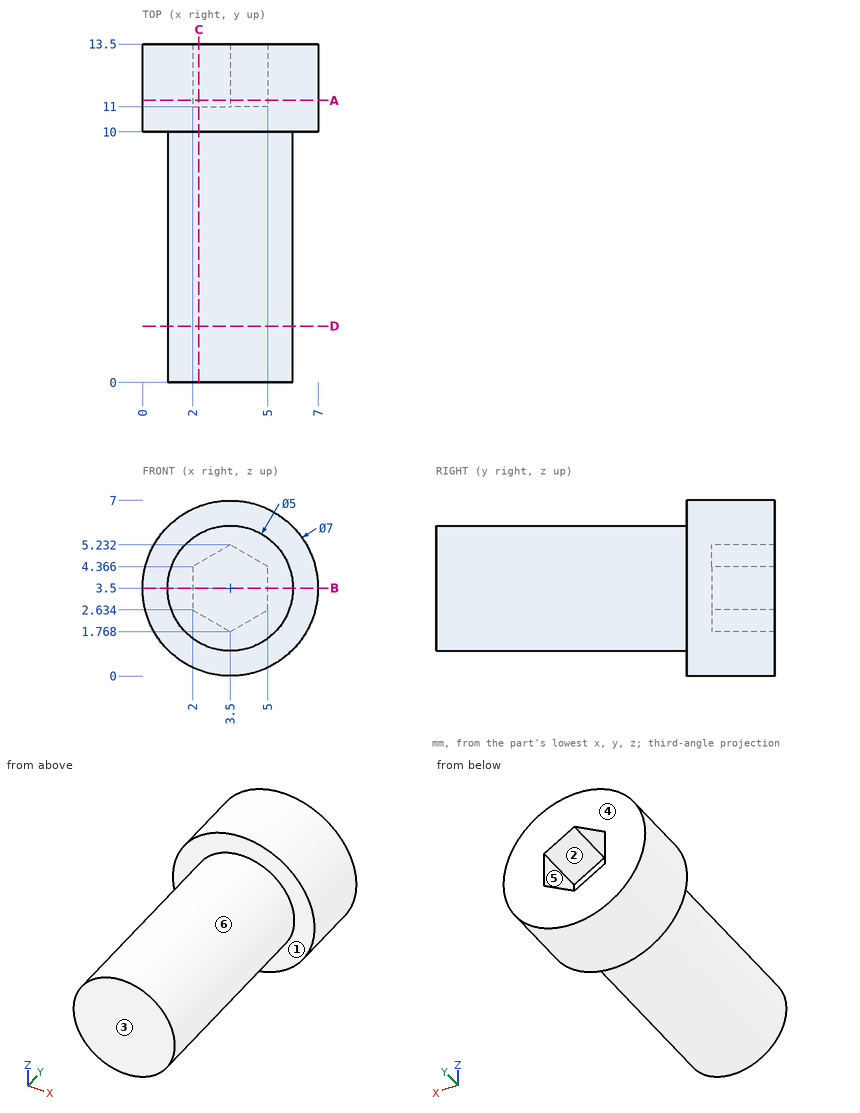
Part print with two shaded views. Sizes in mm from the minimum x, y, z corner. A direction names the side the tool comes from. Round coordinates to 2 decimals unless told otherwise and drop trailing zeros. Order: outer loops, then holes, each group sorted by start corner. A loop starts at its lowest first (then second) coordinate and runs counter-clockwise, first axis right, second up. Notation, with made-up numbers: (-10, 10) - (36, 10) arc R35 ccw to (36, 42) - close; hole circle Ø1 at (34.5, 68). An arc over 180 degrees is marked (long way). Return JSON: item names as keys, results as strings.
(1) Cut at B-B (z = 3.5). Give the cut face in (x, y), then the cut area to 3 significant figures.
Answer key:
{"outline": "(0, 10) - (1, 10) - (1, 0) - (6, 0) - (6, 10) - (7, 10) - (7, 13.5) - (5, 13.5) - (5, 11) - (2, 11) - (2, 13.5) - (0, 13.5) - close", "area": "67.0 mm^2"}
(2) Cut at A-A (y = 11.25). Give the cut face in (x, z).
Answer key:
{"outline": "circle Ø7 at (3.5, 3.5); hole (2, 2.63) - (3.5, 1.77) - (5, 2.63) - (5, 4.37) - (3.5, 5.23) - (2, 4.37) - close"}
(3) Tool access for the marked faces 1, 2 and 3: list every direction of +Z, -Z, +X, -X, +Y, -Y with a clear straight run to the whole face (end or side of a thin tool).
Answer key:
{"face 1": "-Y", "face 2": "+Y", "face 3": "+Z, -Z, +X, -X, -Y"}
(4) Wall check: probe 1 along Y at (x, z) = (1, 5); probe 2 along Y at (x, z) = (3, 4); probe 3 along Z at (x, y) = (5.5, 9). Give the ranges that are in metal, low to high. Write a range as from..to.
Answer key:
{"probe 1": "y = 10..13.5", "probe 2": "y = 0..11", "probe 3": "z = 2..5"}
(5) Pull direction X, two halves, no side cores. Call the marked faces 4, 5 and 6: +X half, -X half, draft (parallel to the pull), parting line (faces both ways), or undercut.
Answer key:
{"face 4": "draft", "face 5": "undercut", "face 6": "parting line"}
(6) Cut at C-C (x = 2.25). Give the cut face in (y, z) (1 decimal).
Answer key:
{"outline": "(0, 1.3) - (10, 1.3) - (10, 0.2) - (13.5, 0.2) - (13.5, 2.5) - (11, 2.5) - (11, 4.5) - (13.5, 4.5) - (13.5, 6.8) - (10, 6.8) - (10, 5.7) - (0, 5.7) - close"}
(7) Pin check, flat tips, straight feed: pin 1 Ø2 at (y, z) = (8, 3) entering from -X; pin 2 Ø0.9 at (x, z) = (3, 3.5) entering from +Y. Stop position of each tip, or through.
Answer key:
{"pin 1": "stops at x = 1", "pin 2": "stops at y = 11"}
(8) Cut at D-D (y = 2.25). Give the cut face in (x, z), then the cut area to 3 significant figures.
Answer key:
{"outline": "circle Ø5 at (3.5, 3.5)", "area": "19.6 mm^2"}
